Build history of the part. All positions in model axes, mm. Face numbers are marked on the shaded views. Give positions to 0.01 mm unless a question says otherwise; leave off trailing zeros. Order: outer loops, then holes, each group sorted by start corner. A loop starts at its lowest first (then second) coordinate and runs counter-clockwise, first axis right, second up. Notation, with made-up numbers: M 54,41 L 103,41 A22 cw 103,52 Z; hole C 19.25,-20.75 d1. An arc over 180 degrees is marked long. One line per item, written item: value. Start each with the question number.
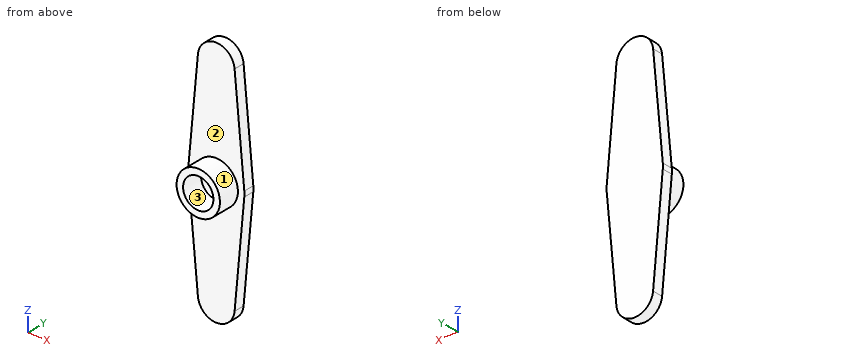
from build123d import *

# Parameters (mm, degrees)
SKETCH_1_R      = 4.25
SKETCH_1_R_2    = 6.5
EXTRUDE_1_DEPTH = 2.5
SKETCH_2_R      = 5
SKETCH_2_R_2    = 3.5
EXTRUDE_2_DEPTH = 5


with BuildPart() as part:
    # 스케치1 → 보스-돌출1 (new body)
    with BuildSketch(Plane(origin=(0, 0, 0), x_dir=(1, 0, 0), z_dir=(0, 1, 0))):
        with BuildLine():
            ThreePointArc((4.25, 24.25), (-0.19737792, 20.004585773), (-4.231666803, 24.644329897))
            Line((-4.231666803, 24.644329897), (-6.471960993, 0.603092784))
            ThreePointArc((-6.471960993, 0.603092784), (0, 6.5), (6.471960993, 0.603092784))
            Line((6.471960993, 0.603092784), (4.231666803, 24.644329897))
            ThreePointArc((4.231666803, 24.644329897), (4.245414227, 24.44737792), (4.25, 24.25))
        make_face()
        with Locations((0, 24.25)):
            Circle(SKETCH_1_R)
        Circle(SKETCH_1_R_2)
        with BuildLine():
            ThreePointArc((6.471960993, -0.603092784), (0, -6.5), (-6.471960993, -0.603092784))
            Line((-6.471960993, -0.603092784), (-4.231666803, -24.644329897))
            ThreePointArc((-4.231666803, -24.644329897), (-0.19737792, -20.004585773), (4.25, -24.25))
            ThreePointArc((4.25, -24.25), (4.245414227, -24.44737792), (4.231666803, -24.644329897))
            Line((4.231666803, -24.644329897), (6.471960993, -0.603092784))
        make_face()
        with Locations((0, -24.25)):
            Circle(SKETCH_1_R)
    extrude(amount=EXTRUDE_1_DEPTH)

    # 스케치2 → 보스-돌출2 (add)
    with BuildSketch(Plane.XZ):
        with Locations(Location((0, 0, 0), (0, 0, 90))):
            Circle(SKETCH_2_R)
        with Locations(Location((0, 0, 0), (0, 0, 270))):
            Circle(SKETCH_2_R_2, mode=Mode.SUBTRACT)
    extrude(amount=EXTRUDE_2_DEPTH)


solid = part.part
1) Drop a flat-ended pin along its axis: P1, Ø5.5, axis at x = 0, z = 0, coming from the -Y side. Give the stop position or say it passes through.
2) Slice it at B-B (y = 1.5). List the corners of the cut face in (x, z).
3) Slice it at C-C (z = 0). List the corners of the cut face in (x, y).
4) Pull direction X, two halves, no side cores. Call the marked faces 1, 2 and 3: pulls with the +X half, pulls with the -X half, needs draft (parallel to the pull), parting line crosses it, or undercut.
5) Slice it at D-D (y = -2). List the corners of the cut face in (x, z).
6) Drill centre lines: line 1 (X direction, y = -1.75, z = 0); line 2 (Y direction, x = 4.5, z = -7); line 3 (Z direction, x = 1.5, y = -1). Where is each one in solid material? Low to high.
7) Slice it at A-A (x = 0). List the corners of the cut face in (y, z).
Results list:
1. P1: stops at y = 0
2. outline: M -6.47,-0.6 L -4.23,-24.64 A4.25 ccw 4.23,-24.64 L 6.47,-0.6 A6.5 ccw 6.47,0.6 L 4.23,24.64 A4.25 ccw -4.23,24.64 L -6.47,0.6 A6.5 ccw Z
3. outline: M -6.5,0 L -5,0 L -5,-5 L -3.5,-5 L -3.5,0 L 3.5,0 L 3.5,-5 L 5,-5 L 5,0 L 6.5,0 L 6.5,2.5 L -6.5,2.5 Z
4. face 1: parting line crosses it
4. face 2: needs draft
4. face 3: undercut
5. outline: C 0,0 d10; hole C 0,0 d7
6. line 1: x = -5 to -3.5, 3.5 to 5
6. line 2: y = 0 to 2.5
6. line 3: z = -4.77 to -3.16, 3.16 to 4.77
7. outline: M -5,-5 L 0,-5 L 0,-28.5 L 2.5,-28.5 L 2.5,28.5 L 0,28.5 L 0,5 L -5,5 L -5,3.5 L 0,3.5 L 0,-3.5 L -5,-3.5 Z
